Design review of the part built by this model. Coordinates are the model's own, in mm. Face numbers are marked on the shaded views. A direction names the side the tool comes from. Give positions to 0.01 mm unless a question says otherwise; leave off trailing zeros. Write each loop counter-clockwise with the first axis right and the second up, starting at its lowest first coordinate (ties: lowest second). Pieces come first, ordered by that corner, then holes. Notation, with made-up numbers: (41, -35.5) - (96, -35.5) arc R21 cw to (96, -29.5) - close; hole circle Ø11 at (88, 85.5). An arc over 180 degrees is marked (long way). Use a Markdown table: item, result. Add a question column.
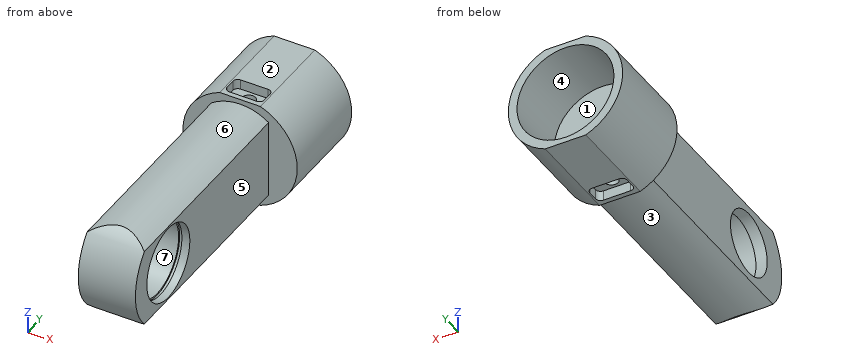
```python
from build123d import *

# Parameters (mm, degrees)
F1_DEPTH  = 38
F3_DEPTH  = 93
F5_DEPTH  = 34.501
F6_R      = 19.5
F7_DEPTH  = 26
F8_R      = 15
F9_DEPTH  = 3.2
F10_R     = 15.7
F11_DEPTH = 1.3
F12_R     = 15
F13_DEPTH = 14
F14_R     = 12.8
F15_DEPTH = 16.001
F17_DEPTH = 4
F19_D     = 5.5
F19_DEPTH = 10
F19_TIP   = 1.6523667023
F21_DEPTH = 4
F23_D     = 5.5
F23_DEPTH = 8.2
F23_TIP   = 1.6523667023


with BuildPart() as f1:
    # F0 (on Front) → F1 (new body)
    with BuildSketch(Plane.XZ):
        with BuildLine():
            Line((8.1700673192, 21.5), (-8.1700673192, 21.5))
            ThreePointArc((-8.1700673192, 21.5), (-23, 0), (-8.1700673192, -21.5))
            Line((-8.1700673192, -21.5), (8.1700673192, -21.5))
            ThreePointArc((8.1700673192, -21.5), (23, 0), (8.1700673192, 21.5))
        make_face()
    extrude(amount=F1_DEPTH)

    # F2 (on face) → F3 (join)
    with BuildSketch(Plane.XZ.offset(38)):
        with BuildLine():
            Line((-11.5, 15.748015748), (-11.5, -15.748015748))
            ThreePointArc((-11.5, -15.748015748), (0, -19.5), (11.5, -15.748015748))
            Line((11.5, -15.748015748), (11.5, 15.748015748))
            ThreePointArc((11.5, 15.748015748), (0, 19.5), (-11.5, 15.748015748))
        make_face()
    extrude(amount=F3_DEPTH)

    # F4 (on face) → F5 (cut, through all)
    with BuildSketch(Plane.YZ.offset(11.5)):
        with BuildLine():
            Line((-108.4063023692, 22.9964109892), (-107.5936976308, 22.9964109892))
            ThreePointArc((-107.5936976308, 22.9964109892), (-108, 23), (-108.4063023692, 22.9964109892))
        make_face()
        with BuildLine():
            ThreePointArc((-110.9123462287, -22.8148688237), (-130.9656634273, 1.256305435), (-108.4063023692, 22.9964109892))
            Line((-108.4063023692, 22.9964109892), (-137.5913057301, 22.9964109892))
            Line((-137.5913057301, 22.9964109892), (-137.5913057301, -22.410525009))
            Line((-137.5913057301, -22.410525009), (-110.9123462287, -22.8148688237))
        make_face()
    extrude(amount=-F5_DEPTH, mode=Mode.SUBTRACT)

    # F6 (on face) → F7 (cut)
    with BuildSketch(Plane(origin=(0, 0, 0), x_dir=(-1, 0, 0), z_dir=(0, 1, 0))):
        Circle(F6_R)
    extrude(amount=-F7_DEPTH, mode=Mode.SUBTRACT)

    # F8 (on face) → F9 (cut)
    with BuildSketch(Plane.YZ.offset(11.5)):
        with Locations((-108, 0)):
            Circle(F8_R)
    extrude(amount=-F9_DEPTH, mode=Mode.SUBTRACT)

    # F10 (on face) → F11 (cut)
    with BuildSketch(Plane.YZ.offset(8.3)):
        with Locations((-108, 0)):
            Circle(F10_R)
    extrude(amount=-F11_DEPTH, mode=Mode.SUBTRACT)

    # F12 (on face) → F13 (cut)
    with BuildSketch(Plane.YZ.offset(7)):
        with Locations((-108, 0)):
            Circle(F12_R)
    extrude(amount=-F13_DEPTH, mode=Mode.SUBTRACT)

    # F14 (on face) → F15 (cut, through all)
    with BuildSketch(Plane.YZ.offset(-7)):
        with Locations((-108, 0)):
            Circle(F14_R)
    extrude(amount=-F15_DEPTH, mode=Mode.SUBTRACT)

    # F16 (on face) → F17 (cut)
    with BuildSketch(Plane.XY.offset(21.5)):
        with BuildLine():
            Line((5.5, -28), (-5.5, -28))
            ThreePointArc((-5.5, -28), (-6.9142135624, -28.5857864376), (-7.5, -30))
            Line((-7.5, -30), (-7.5, -34))
            ThreePointArc((-7.5, -34), (-6.9142135624, -35.4142135624), (-5.5, -36))
            Line((-5.5, -36), (5.5, -36))
            ThreePointArc((5.5, -36), (6.9142135624, -35.4142135624), (7.5, -34))
            Line((7.5, -34), (7.5, -30))
            ThreePointArc((7.5, -30), (6.9142135624, -28.5857864376), (5.5, -28))
        make_face()
    extrude(amount=-F17_DEPTH, mode=Mode.SUBTRACT)

    # F19
    with Locations(Plane.XY.offset(17.5)):
        with Locations((0, -32)):
            Hole(F19_D / 2, depth=F19_DEPTH)
            with Locations((0, 0, -(F19_DEPTH + F19_TIP / 2))):  # 118° drill point
                Cone(0, F19_D / 2, F19_TIP, mode=Mode.SUBTRACT)

    # F20 (on face) → F21 (cut)
    with BuildSketch(Plane(origin=(0, 0, -21.5), x_dir=(1, 0, 0), z_dir=(0, 0, -1))):
        with BuildLine():
            Line((5.5, 36), (-5.5, 36))
            ThreePointArc((-5.5, 36), (-6.9142135624, 35.4142135624), (-7.5, 34))
            Line((-7.5, 34), (-7.5, 30))
            ThreePointArc((-7.5, 30), (-6.9142135624, 28.5857864376), (-5.5, 28))
            Line((-5.5, 28), (5.5, 28))
            ThreePointArc((5.5, 28), (6.9142135624, 28.5857864376), (7.5, 30))
            Line((7.5, 30), (7.5, 34))
            ThreePointArc((7.5, 34), (6.9142135624, 35.4142135624), (5.5, 36))
        make_face()
    extrude(amount=-F21_DEPTH, mode=Mode.SUBTRACT)

    # F23
    with Locations(Plane(origin=(0, 0, -17.5), x_dir=(1, 0, 0), z_dir=(0, 0, -1))):
        with Locations((0, 32)):
            Hole(F23_D / 2, depth=F23_DEPTH)
            with Locations((0, 0, -(F23_DEPTH + F23_TIP / 2))):  # 118° drill point
                Cone(0, F23_D / 2, F23_TIP, mode=Mode.SUBTRACT)


solid = f1.part
```
(1) Insertion check: pin 1 (3 mm diameter, centred on x = -11, z = 6, fed in from +Y); pin 2 (4 mm diameter, centred on x = 5, y = -30.5, fed in from +Z); pin 3 (1.5 mm diameter, centred on x = -16, y = -31.5, fed in from -Z); pin 4 (1.2 mm diameter, centred on x = 2.5, z = -20.5, fed in from +Y). Each pin has a flat end and moves straight along its axis. Give the tip position at first contact, or say it passes through.
(2) Add section C-C (y = -18). State the section outline as (x, z) points.
(3) Add section B-B (x = 13). State the section outline as (y, z) points, and give its area (3 significant figures).
(4) Add section A-A (y = -108). State the section outline as (x, z) points.
(5) For line 1 along Z through (x, y) = (0, -8); line 2 along Z through (x, y) = (9.5, -18.5); line 3 along X through (y, z) = (-74, -11.5), list the stretches that pass through material, from the lowest coordinate up.
(6) Add section D-D (y = -71). State the section outline as (x, z) points.
(7) Tool access review of the marked faces 5, 6 and 7: name each direction out of +Z, -Z, +X, -X, +Y, -Y from which nothing blocks a thin tool from reaching the whole face with its end or side.
(8) Mouldability with a two-part tool opening along Z and no side actions: class the marked faces 1, 2, 3 and 4 as +Z half, -Z half, draft (parallel to the pull), parting line (faces both ways), or undercut.
Answers follow:
| question | item | result |
|---|---|---|
| 1 | pin 1 | y = -26 |
| 1 | pin 2 | z = 17.5 |
| 1 | pin 3 | z = -17.22 |
| 1 | pin 4 | y = 0 |
| 2 | outline | (-8.17, -21.5) - (8.17, -21.5) arc R23 ccw to (8.17, 21.5) - (-8.17, 21.5) arc R23 ccw to start; hole circle Ø39 at (0, 0) |
| 3 | outline | (-38, -18.97) - (0, -18.97) - (0, -14.53) - (-26, -14.53) - (-26, 14.53) - (0, 14.53) - (0, 18.97) - (-38, 18.97) - close |
| 3 | area | 686 mm^2 |
| 4 | outline | (-11.5, -15.75) arc R19.5 ccw to (11.5, -15.75) - (11.5, -15) - (8.3, -15) - (8.3, -15.7) - (7, -15.7) - (7, -15) - (-7, -15) - (-7, -12.8) - (-11.5, -12.8) - close; (-11.5, 12.8) - (-7, 12.8) - (-7, 15) - (7, 15) - (7, 15.7) - (8.3, 15.7) - (8.3, 15) - (11.5, 15) - (11.5, 15.75) arc R19.5 ccw to (-11.5, 15.75) - close |
| 5 | line 1 | -21.5 to -19.5, 19.5 to 21.5 |
| 5 | line 2 | -20.95 to -17.03, 17.03 to 20.95 |
| 5 | line 3 | -11.5 to 11.5 |
| 6 | outline | (-11.5, -15.75) arc R19.5 ccw to (11.5, -15.75) - (11.5, 15.75) arc R19.5 ccw to (-11.5, 15.75) - close |
| 7 | face 5 | +Z, -Z, +X, -Y |
| 7 | face 6 | +Z, -Y |
| 7 | face 7 | +X |
| 8 | face 1 | undercut |
| 8 | face 2 | +Z half |
| 8 | face 3 | -Z half |
| 8 | face 4 | undercut |
